```python
from build123d import *

# Parameters (mm, degrees)
SKETCH1_W                  = 298.45
SKETCH1_H                  = 495.3
BOSS_EXTRUDE1_DEPTH        = 4.7625
CUT_EXTRUDE1_DEPTH         = 290.291114191
CUT_EXTRUDE1_DEPTH_BACK    = 290.291114191
SKETCH3_W                  = 196.85
SKETCH3_H                  = 114.3
SKETCH20_W                 = 47.879
SKETCH20_H                 = 47.879
CUT_EXTRUDE5_DEPTH         = 290.291114191
F_10_CLEARANCE_HOLE1_D     = 5.1054
F_10_CLEARANCE_HOLE1_DEPTH = 10.668
F_10_CLEARANCE_HOLE1_TIP   = 1.533816902
F_10_CLEARANCE_HOLE4_D     = 5.1054
LPATTERN3_COUNT            = 3
LPATTERN3_PITCH            = 63.5
MIRROR2_COPY_1_D           = 5.1054
MIRROR2_COPY_2_D           = 5.1054
F_10_CLEARANCE_HOLE5_D     = 5.1054
LPATTERN4_COUNT            = 3
LPATTERN4_PITCH            = 96.52
LPATTERN4_COL_COUNT        = 3
LPATTERN4_COL_PITCH        = 96.52
MIRROR3_COPY_1_D           = 5.1054
MIRROR3_COPY_2_D           = 5.1054
MIRROR3_COPY_3_D           = 5.1054
MIRROR3_COPY_4_D           = 5.1054
F_10_CLEARANCE_HOLE6_D     = 5.1054
F_10_CLEARANCE_HOLE7_D     = 5.1054
F_1_4_20_TAPPED_HOLE1_D    = 5.1054


with BuildPart() as part:
    # Sketch1 → Boss-Extrude1 (new, symmetric)
    with BuildSketch(Plane(origin=(0, 0, 0), x_dir=(1, 0, 0), z_dir=(0, 1, 0))):
        Rectangle(SKETCH1_W, SKETCH1_H)
    extrude(amount=BOSS_EXTRUDE1_DEPTH, both=True)

    # Sketch3 → Cut-Extrude1 (cut, two sides: drawn at the far end of the back side and taken through both)
    with BuildSketch(Plane(origin=(0, 4.7625, 0), x_dir=(1, 0, 0), z_dir=(0, 1, 0)).offset(-CUT_EXTRUDE1_DEPTH_BACK)):
        with Locations((0, -44.45)):
            Rectangle(SKETCH3_W, SKETCH3_H)
    extrude(amount=CUT_EXTRUDE1_DEPTH + CUT_EXTRUDE1_DEPTH_BACK, mode=Mode.SUBTRACT)

    # Sketch20 → Cut-Extrude5 (cut, through all)
    with BuildSketch(Plane.XZ.offset(4.7625)):
        with Locations((0, 171.45)):
            Rectangle(SKETCH20_W, SKETCH20_H)
    extrude(amount=-CUT_EXTRUDE5_DEPTH, mode=Mode.SUBTRACT)

    # #10 Clearance Hole1
    with Locations(Plane(origin=(0, -4.7625, 0), x_dir=(-1, 0, 0), z_dir=(0, -1, 0))):
        with Locations((-38.1, -155.575), (38.1, -155.575), (38.1, -187.325), (-38.1, -187.325)):
            Hole(F_10_CLEARANCE_HOLE1_D / 2, depth=F_10_CLEARANCE_HOLE1_DEPTH)
            with Locations((0, 0, -(F_10_CLEARANCE_HOLE1_DEPTH + F_10_CLEARANCE_HOLE1_TIP / 2))):  # 118° drill point
                Cone(0, F_10_CLEARANCE_HOLE1_D / 2, F_10_CLEARANCE_HOLE1_TIP, mode=Mode.SUBTRACT)

    # #10 Clearance Hole4 (through all)
    with Locations(Plane(origin=(0, 4.7625, 0), x_dir=(1, 0, 0), z_dir=(0, 1, 0))):
        with Locations((-63.5, 241.3)):
            f_10_clearance_hole4 = Hole(F_10_CLEARANCE_HOLE4_D / 2)

    # LPattern3: #10 Clearance Hole4 ×3
    with Locations(*[(i * LPATTERN3_PITCH, 0, 0) for i in range(1, LPATTERN3_COUNT)]):
        add(f_10_clearance_hole4, mode=Mode.SUBTRACT)

    # Mirror2: #10 Clearance Hole4 across plane
    add(f_10_clearance_hole4.mirror(Plane.XY), mode=Mode.SUBTRACT)

    # Mirror2 copy 1 (through all)
    with Locations(Plane(origin=(63.5, 4.7625, 0), x_dir=(1, 0, 0), z_dir=(0, 1, 0))):
        with Locations((-63.5, -241.3)):
            Hole(MIRROR2_COPY_1_D / 2)

    # Mirror2 copy 2 (through all)
    with Locations(Plane(origin=(127, 4.7625, 0), x_dir=(1, 0, 0), z_dir=(0, 1, 0))):
        with Locations((-63.5, -241.3)):
            Hole(MIRROR2_COPY_2_D / 2)

    # #10 Clearance Hole5 (through all)
    with Locations(Plane(origin=(0, 4.7625, 0), x_dir=(1, 0, 0), z_dir=(0, 1, 0))):
        with Locations((-142.875, 0)):
            f_10_clearance_hole5 = Hole(F_10_CLEARANCE_HOLE5_D / 2)

    # LPattern4: #10 Clearance Hole5 ×3
    with Locations(*[(0, 0, -i * LPATTERN4_PITCH) for i in range(1, LPATTERN4_COUNT)]):
        add(f_10_clearance_hole5, mode=Mode.SUBTRACT)

    # LPattern4 col: #10 Clearance Hole5 ×3
    with Locations(*[(0, 0, i * LPATTERN4_COL_PITCH) for i in range(1, LPATTERN4_COL_COUNT)]):
        add(f_10_clearance_hole5, mode=Mode.SUBTRACT)

    # Mirror3: #10 Clearance Hole5 across plane
    add(f_10_clearance_hole5.mirror(Plane(origin=(0, 0, 0), x_dir=(0, 0, 1), z_dir=(1, 0, 0))), mode=Mode.SUBTRACT)

    # Mirror3 copy 1 (through all)
    with Locations(Plane(origin=(0, 4.7625, -96.52), x_dir=(-1, 0, 0), z_dir=(0, 1, 0))):
        with Locations((-142.875, 0)):
            Hole(MIRROR3_COPY_1_D / 2)

    # Mirror3 copy 2 (through all)
    with Locations(Plane(origin=(0, 4.7625, -193.04), x_dir=(-1, 0, 0), z_dir=(0, 1, 0))):
        with Locations((-142.875, 0)):
            Hole(MIRROR3_COPY_2_D / 2)

    # Mirror3 copy 3 (through all)
    with Locations(Plane(origin=(0, 4.7625, 96.52), x_dir=(-1, 0, 0), z_dir=(0, 1, 0))):
        with Locations((-142.875, 0)):
            Hole(MIRROR3_COPY_3_D / 2)

    # Mirror3 copy 4 (through all)
    with Locations(Plane(origin=(0, 4.7625, 193.04), x_dir=(-1, 0, 0), z_dir=(0, 1, 0))):
        with Locations((-142.875, 0)):
            Hole(MIRROR3_COPY_4_D / 2)

    # #10 Clearance Hole6 (through all)
    with Locations(Plane(origin=(0, 4.7625, 0), x_dir=(1, 0, 0), z_dir=(0, 1, 0))):
        with Locations((120.65, 32.5755), (120.65, -121.4755), (-120.65, -121.4755), (-120.65, 32.5755)):
            Hole(F_10_CLEARANCE_HOLE6_D / 2)

    # #10 Clearance Hole7 (through all)
    with Locations(Plane(origin=(0, 4.7625, 0), x_dir=(1, 0, 0), z_dir=(0, 1, 0))):
        with Locations((76.2, 32.5755), (0, 32.5755), (-76.2, 32.5755), (76.2, -121.4755), (0, -121.4755), (-76.2, -121.4755)):
            Hole(F_10_CLEARANCE_HOLE7_D / 2)

    # 1/4-20 Tapped Hole1 (through all)
    with Locations(Plane(origin=(0, 4.7625, 0), x_dir=(1, 0, 0), z_dir=(0, 1, 0))):
        with Locations((-128.905, -44.45), (128.905, -44.45)):
            Hole(F_1_4_20_TAPPED_HOLE1_D / 2)


solid = part.part
```
The model under review builds one solid part; all positions refer to its coordinate system, in mm. A direction names the side the tool comes from. Round coordinates to 2 decimals unless told otherwise and drop trailing zeros. Order: outer loops, then holes, each group sorted by start corner. A loop starts at its lowest first (then second) coordinate and runs counter-clockwise, first axis right, second up.
Item 1: To check wall thickness, follow probe 1 along Z at (x, y) = (-18, -2.5); probe 2 along X at (y, z) = (-2.5, -241.3) (3 decimals); probe 3 along X at (y, z) = (-0.5, 193.04) (1 decimal). State the ranges of each line that lie inside material, in increasing order.
Working result:
probe 1: z = -247.65 to -12.7, 101.6 to 147.51, 195.39 to 247.65
probe 2: x = -149.225 to -66.053, -60.947 to -2.553, 2.553 to 60.947, 66.053 to 149.225
probe 3: x = -149.2 to -145.4, -140.3 to -23.9, 23.9 to 140.3, 145.4 to 149.2
Item 2: Machinability: for faces 1 (the flat face through (-2, -4.762, -59)), 2 (the flat face through (0, 0, 195.39)), which of the approach directions +Z, -Z, +X, -X, +Y, -Y give a long, thin tool a straight path to every point of the face, cutting with its end or side? Answer none if there is none.
Working result:
face 1: +Z, -Z, +X, -X, -Y
face 2: +Y, -Y
Item 3: Add section B-B, the plane y = -3.25. Count the separate pieces of the cut face and the enclosed holes in it, and give its area (3 significant figures).
Working result:
separate pieces: 1
enclosed holes: 34
area: 122,000 mm2
Item 4: Draft analysis for pull direction X (two halves, no side actions). For faces 3 (the flat face through (-2, 0, 247.65)), 4 (the flat face through (-98.425, 0, 45)), 5 (the flat face through (-149.225, 0, 3)), state which applies: released by +X, released by -X, zero draft, split by the parting line, or undercut.
Working result:
face 3: zero draft
face 4: undercut
face 5: released by -X
Item 5: For pin 1 (4.5 mm diameter, centred on x = -38.1, z = 187.325, fed in from +Y), flat-tipped, find the tip position at first contact; note if it passes through.
Working result:
pin 1: passes through
Item 6: Add section A-A, the plane x = 30.5. State the section outline as (y, z) points.
Working result:
outline: (-4.76, -247.65) - (4.76, -247.65) - (4.76, -12.7) - (-4.76, -12.7) - close; (-4.76, 101.6) - (4.76, 101.6) - (4.76, 247.65) - (-4.76, 247.65) - close
